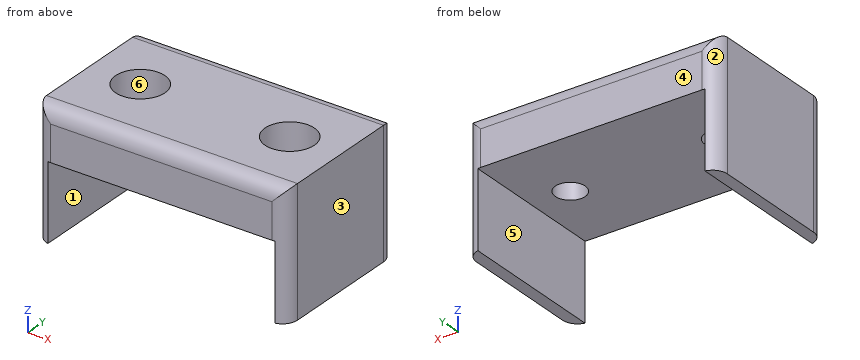
```python
from build123d import *

# Parameters (mm, degrees)
BOSS_EXTRUDE1_DEPTH = 25.4
SKETCH2_R           = 2.54
CUT_EXTRUDE1_DEPTH  = 40.579199032
SKETCH3_R           = 4.191
CUT_EXTRUDE2_DEPTH  = 5.08
FILLET1_R           = 2.54
FILLET2_R           = 2.54


with BuildPart() as part:
    # Sketch1 → Boss-Extrude1 (new body)
    with BuildSketch(Plane(origin=(0, 0, 0), x_dir=(1, 0, 0), z_dir=(0, 1, 0))):
        Polygon((-19.304, 0), (-21.336, 0), (-21.336, -21.59), (21.336, -21.59), (21.336, 0), (19.304, 0), (19.304, -12.954), (-19.304, -12.954), align=None)
    extrude(amount=BOSS_EXTRUDE1_DEPTH)

    # Sketch2 → Cut-Extrude1 (cut, through all)
    with BuildSketch(Plane.XY.offset(21.59)):
        with Locations((-12.7, 12.7)):
            Circle(SKETCH2_R)
        with Locations((12.7, 12.7)):
            Circle(SKETCH2_R)
    extrude(amount=-CUT_EXTRUDE1_DEPTH, mode=Mode.SUBTRACT)

    # Sketch3 → Cut-Extrude2 (cut)
    with BuildSketch(Plane.XY.offset(21.59)):
        with Locations((-12.7, 12.7)):
            Circle(SKETCH3_R)
        with Locations((12.7, 12.7)):
            Circle(SKETCH3_R)
    extrude(amount=-CUT_EXTRUDE2_DEPTH, mode=Mode.SUBTRACT)

    # Fillet1
    fillet1_edges = [part.edges().sort_by_distance(p)[0] for p in [
        (-21.336, 25.4, 10.795),
        (21.336, 25.4, 10.795),
        (0, 25.4, 21.59),
    ]]
    fillet(fillet1_edges, radius=FILLET1_R)

    # Fillet2
    fillet2_edges = [part.edges().sort_by_distance(p)[0] for p in [
        (-21.336, 0, 10.795),
        (0, 0, 21.59),
        (21.336, 0, 10.795),
    ]]
    fillet(fillet2_edges, radius=FILLET2_R)


solid = part.part
```
Geometry: final body of the model. Coordinates: model frame, mm. Face numbers are marked on the shaded views. A direction names the side the tool comes from. Coordinates: 2 decimals unless noted, no trailing zeros. Order: outer loops, then holes, each group sorted by start corner. A loop starts at its lowest first (then second) coordinate and runs counter-clockwise, first axis right, second up. Notation, with made-up numbers: M 61,31 L 87,31 A21 cw 87,55 Z; hole C 63.25,-23.5 d7. An arc over 180 degrees is marked long. Answer in a Markdown table with one row per item. Add a question column.
Q1. Contact query for flat-ended pins moving along their axis: P1, Ø4, axis at x = -12.5, y = 13.5, coming from the +Z side; P2, Ø7.5, axis at x = -5.5, y = 13.5, coming from the -Z side. Output: stop coordinate, or through.
Q2. Section query C-C on y = 12.7. Return the cut outline in (x, z), and give its area (3 significant figures).
Q3. Section query B-B on x = -12.7. Return the cut outline in (y, z).
Q4. Line query: L1, parallel to Y at x = -12.7, z = 14.85; L2, parallel to X at y = 8.5, z = 7.25; L3, parallel to Y at x = 12.7, z = 18.15. Output: solid intervals per line, ascending.
Q5. Mould query, pull axis X, two halves, no side actions, for the marked faces 1, 2 and 3. Classes: released by +X, released by -X, zero draft, split by the parting line, or undercut.
Q6. Section query A-A on z = 12.5. Return the cut outline in (x, y), and give its area (3 significant figures).
Q7. Section query D-D on y = 7.25. Return the cut outline in (x, z), and give its area (3 significant figures).
Q8. Reachability of the marked faces 4, 5 and 6 from +Z, -Z, +X, -X, +Y, -Y: full face, straight path, thin tool, end or side. Return the list, or none.
Completed:
| question | item | result |
|---|---|---|
| 1 | P1 | stops at z = 16.51 |
| 1 | P2 | stops at z = 12.95 |
| 2 | outline | M -21.34,0 L -19.3,0 L -19.3,12.95 L -15.24,12.95 L -15.24,16.51 L -16.89,16.51 L -16.89,21.59 L -21.34,21.59 Z; M -10.16,12.95 L 10.16,12.95 L 10.16,16.51 L 8.51,16.51 L 8.51,21.59 L -8.51,21.59 L -8.51,16.51 L -10.16,16.51 Z; M 15.24,12.95 L 19.3,12.95 L 19.3,0 L 21.34,0 L 21.34,21.59 L 16.89,21.59 L 16.89,16.51 L 15.24,16.51 Z |
| 2 | area | 300 mm2 |
| 3 | outline | M 0,12.95 L 10.16,12.95 L 10.16,16.51 L 8.51,16.51 L 8.51,21.59 L 2.54,21.59 A2.54 ccw 0,19.05 Z; M 15.24,12.95 L 25.4,12.95 L 25.4,19.05 A2.54 ccw 22.86,21.59 L 16.89,21.59 L 16.89,16.51 L 15.24,16.51 Z |
| 4 | L1 | y = 0 to 10.16, 15.24 to 25.4 |
| 4 | L2 | x = -21.34 to -19.3, 19.3 to 21.34 |
| 4 | L3 | y = 0 to 8.51, 16.89 to 25.4 |
| 5 | face 1 | undercut |
| 5 | face 2 | released by -X |
| 5 | face 3 | released by +X |
| 6 | outline | M -21.34,2.54 A2.54 ccw -19.3,0.05 L -19.3,25.35 A2.54 ccw -21.34,22.86 Z; M 19.3,0.05 A2.54 ccw 21.34,2.54 L 21.34,22.86 A2.54 ccw 19.3,25.35 Z |
| 6 | area | 97.7 mm2 |
| 7 | outline | M -21.34,0 L -19.3,0 L -19.3,12.95 L 19.3,12.95 L 19.3,0 L 21.34,0 L 21.34,21.59 L -21.34,21.59 Z |
| 7 | area | 421 mm2 |
| 8 | face 4 | +Z, -Z, +X, -X, +Y |
| 8 | face 5 | -Z, +Y, -Y |
| 8 | face 6 | +Z |
